Read the model definition and answer for the solid it produces. Units are mm, in the model's axes. Give positions to 0.01 mm unless a question says otherwise; leave off trailing zeros. Order: outer loops, then holes, each group sorted by start corner. A loop starts at its lowest first (then second) coordinate and runs counter-clockwise, first axis right, second up. Notation, with made-up numbers: (8, 46) -> (57, 46) arc R29 cw to (57, 76) -> close; hole circle Ø9 at (57.5, -22.75). An arc over 180 degrees is marked (long way). Answer as CSV lines item,"result". Start each with the question number.
1) Find section A-A (z = 18). Determine the outline of the cut face in (x, y) (3 decimals), and give its area (3 significant figures).
2) A flat-ended cylindrical pin translates along its axis: pin 1 Ø8 at (x, z) = (-12.5, 30.5) entering from -Y (3 decimals). Find the tip coordinate at first contact, or state that the pin passes through.
3) Find section C-C (y = -5.25). Determine the outline of the cut face in (x, z), and give its area (3 significant figures).
4) Find section D-D (x = 12.5). Determine the outline of the cut face in (y, z) (3 decimals).
5) The mould has two halves that part along X. Classify faces 1 (the face through (10.29, 0.12, 3.47)), 2 (the face through (18, 0, 18)), 3 (the face through (-14.71, 0.12, 3.47)), 4 (the face through (-8, -8.425, 26)): +X half, -X half, draft (parallel to the pull), parting line (faces both ways), or undercut.
6) Straight lines are drawn through the part: L1, parallel to Z at x = 12.5, y = 4.75; L2, parallel to X at y = -0.5, z = 5.5; L3, parallel to Z at x = -13.5, y = -4.25. For each, find the intervals that lie inside material, in ascending order. Write a range as from..to.
7) Find section B-B (x = -8). Determine the outline of the cut face in (y, z) (3 decimals), and give its area (3 significant figures).
```python
from build123d import *

# Parameters (mm, degrees)
SKETCH_1_W          = 36
SKETCH_1_H          = 16.85
EXTRUDE_1_DEPTH     = 36
SKETCH_2_R          = 3
CUT_EXTRUDE_1_DEPTH = 17.85
SKETCH_3_R          = 10
CUT_EXTRUDE_2_DEPTH = 17.85
FILLET_1_R          = 2


with BuildPart() as part:
    # 草图1 → 凸台-拉伸1 (new body)
    with BuildSketch(Plane.XY):
        Rectangle(SKETCH_1_W, SKETCH_1_H)
    extrude(amount=EXTRUDE_1_DEPTH)

    # 草图2 → 切除-拉伸1 (cut, through all)
    with BuildSketch(Plane(origin=(0, 8.425, 0), x_dir=(1, 0, 0), z_dir=(0, 1, 0))):
        with Locations((-12.5, -5.5)):
            Circle(SKETCH_2_R)
        with Locations((-12.5, -30.5)):
            Circle(SKETCH_2_R)
        with Locations((12.5, -30.5)):
            Circle(SKETCH_2_R)
        with Locations((12.5, -5.5)):
            Circle(SKETCH_2_R)
    extrude(amount=-CUT_EXTRUDE_1_DEPTH, mode=Mode.SUBTRACT)

    # 草图3 → 切除-拉伸2 (cut, through all)
    with BuildSketch(Plane(origin=(0, 8.425, 0), x_dir=(1, 0, 0), z_dir=(0, 1, 0))):
        with Locations((0, -18)):
            Circle(SKETCH_3_R)
    extrude(amount=-CUT_EXTRUDE_2_DEPTH, mode=Mode.SUBTRACT)

    # 圆角1
    fillet_1_edges = [part.edges().sort_by_distance(p)[0] for p in [
        (-18, 0, 36),
        (18, 0, 36),
        (-18, 0, 0),
        (18, 0, 0),
    ]]
    fillet(fillet_1_edges, radius=FILLET_1_R)


solid = part.part
```
Findings below:
1,outline,"(-18, -8.425) -> (-10, -8.425) -> (-10, 8.425) -> (-18, 8.425) -> close; (10, -8.425) -> (18, -8.425) -> (18, 8.425) -> (10, 8.425) -> close"
1,area,"270 mm²"
2,pin 1,"y = -8.425"
3,outline,"(-18, 2) arc R2 ccw to (-16, 0) -> (16, 0) arc R2 ccw to (18, 2) -> (18, 34) arc R2 ccw to (16, 36) -> (-16, 36) arc R2 ccw to (-18, 34) -> close; hole circle Ø6 at (-12.5, 5.5); hole circle Ø6 at (-12.5, 30.5); hole circle Ø20 at (0, 18); hole circle Ø6 at (12.5, 5.5); hole circle Ø6 at (12.5, 30.5)"
3,area,"865 mm²"
4,outline,"(-8.425, 0) -> (8.425, 0) -> (8.425, 2.5) -> (-8.425, 2.5) -> close; (-8.425, 8.5) -> (8.425, 8.5) -> (8.425, 27.5) -> (-8.425, 27.5) -> close; (-8.425, 33.5) -> (8.425, 33.5) -> (8.425, 36) -> (-8.425, 36) -> close"
5,face 1,"undercut"
5,face 2,"+X half"
5,face 3,"undercut"
5,face 4,"draft"
6,L1,"0..2.5, 8.5..27.5, 33.5..36"
6,L2,"-18..-15.5, -9.5..9.5, 15.5..18"
6,L3,"0..2.67, 8.33..27.67, 33.33..36"
7,outline,"(-8.425, 0) -> (8.425, 0) -> (8.425, 12) -> (-8.425, 12) -> close; (-8.425, 24) -> (8.425, 24) -> (8.425, 36) -> (-8.425, 36) -> close"
7,area,"404 mm²"
